Check sheet for the modelled part. Datum: model origin and axes. Units: mm. Coordinates: 2 decimals unless noted, no trailing zeros. Loops run counter-clockwise (first coordinate to the right, second up) from the corner with the lowest first, then second, coordinate; pieces in that order, holes last. Notation, with made-up numbers: M 80.5,75.5 L 93.5,75.5 A33 ccw 93.5,108.5 Z; hole C -17,-22 d10. An arc over 180 degrees is marked long. Use CSV: the item, a comma, the result in double quotes. Start each with the question number.
(1) Go/stop test with flat-tipped pins: pin 1 Ø12 at (y, z) = (-21.5, 27) entering from -X; pin 2 Ø4 at (x, y) = (-55, -19.5) entering from -Z; pin 3 Ø8 at (y, z) = (-11, 32.5) entering from +X. Record where each tip stops, or that it passes through.
(2) Section check C-C on z = 41. Record the cut outline in (x, y), and give its area (3 significant figures).
(3) Section check D-D on y = -23. Record the cut outline in (x, z), and give its area (3 significant figures).
(4) Section check B-B on x = -51. Record the cut outline in (y, z), and give its area (3 significant figures).
(5) Scan lines: line 1 (Z direction, x = -48, y = -13); line 2 (X direction, y = -12.75, z = 47); line 3 (Z direction, x = -43, y = -11). Record each from-to range of solid material in increasing order.
(6) Section check A-A on x = -37.5. Record the cut outline in (y, z), and give its area (3 significant figures).
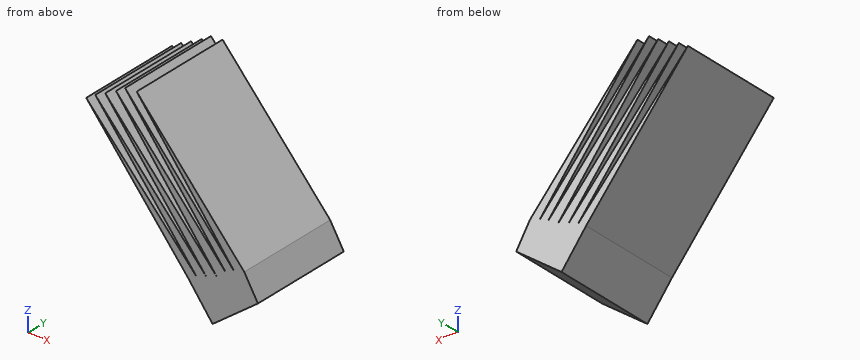
from build123d import *

# Parameters (mm, degrees)
F1_DEPTH = 25.4
F2_DEPTH = 25.4


with BuildPart() as f1:
    # F0 (on Front) → F1 (new body)
    with BuildSketch(Plane.XZ):
        Polygon((-59.2448, 50.682843), (-35.03513, 20.962032), (-29.193482, 13.1901), (-18.408047, 21.296799), (-21.650923, 26.866825), (-47.238376, 56.193985), (-23.816016, 25.882695), (-49.993947, 55.997163), (-25.78428, 24.898561), (-52.159041, 54.619372), (-28.1462, 23.520775), (-54.717787, 53.241584), (-30.704945, 22.733469), (-57.079706, 52.060626), (-32.870036, 21.749334), align=None)
    extrude(amount=F1_DEPTH)

    # F0 (on Front) → F2 (join)
    with BuildSketch(Plane.XZ):
        Polygon((-59.2448, 50.682843), (-35.03513, 20.962032), (-29.193482, 13.1901), (-18.408047, 21.296799), (-21.650923, 26.866825), (-47.238376, 56.193985), (-23.816016, 25.882695), (-49.993947, 55.997163), (-25.78428, 24.898561), (-52.159041, 54.619372), (-28.1462, 23.520775), (-54.717787, 53.241584), (-30.704945, 22.733469), (-57.079706, 52.060626), (-32.870036, 21.749334), align=None)
    extrude(amount=F2_DEPTH)


solid = f1.part
Outcome:
1,pin 1,"stops at x = -44.84"
1,pin 2,"stops at z = 43.02"
1,pin 3,"stops at x = -23.08"
2,outline,"M -51.36,-25.4 L -50.42,-25.4 L -50.42,0 L -51.36,0 Z; M -48.25,-25.4 L -47.13,-25.4 L -47.13,0 L -48.25,0 Z; M -45.08,-25.4 L -43.77,-25.4 L -43.77,0 L -45.08,0 Z; M -41.64,-25.4 L -40.07,-25.4 L -40.07,0 L -41.64,0 Z; M -38.32,-25.4 L -36.96,-25.4 L -36.96,0 L -38.32,0 Z; M -35.5,-25.4 L -33.98,-25.4 L -33.98,0 L -35.5,0 Z"
2,area,"198 mm²"
3,outline,"M -59.24,50.68 L -35.04,20.96 L -29.19,13.19 L -18.41,21.3 L -21.65,26.87 L -47.24,56.19 L -23.82,25.88 L -49.99,56 L -25.78,24.9 L -52.16,54.62 L -28.15,23.52 L -54.72,53.24 L -30.7,22.73 L -57.08,52.06 L -32.87,21.75 Z"
3,area,"385 mm²"
4,outline,"M -25.4,40.56 L 0,40.56 L 0,41.64 L -25.4,41.64 Z; M -25.4,44.45 L 0,44.45 L 0,45.3 L -25.4,45.3 Z; M -25.4,48.52 L 0,48.52 L 0,49.08 L -25.4,49.08 Z; M -25.4,53.12 L 0,53.12 L 0,53.31 L -25.4,53.31 Z"
4,area,"68.3 mm²"
5,line 1,"z = 36.88 to 38.35, 40.69 to 41.96, 44.71 to 45.73, 49.23 to 49.93, 53.44 to 53.7"
5,line 2,"x = -56.24 to -55.89, -53.04 to -52.53, -49.81 to -49.14, -46.28 to -45.4, -42.99 to -42.17, -40.13 to -39.22"
5,line 3,"z = 30.74 to 32.86, 34.43 to 36.4, 38.35 to 40.14, 42.76 to 44.3, 47.01 to 47.95, 50.71 to 51.34"
6,outline,"M -25.4,23.99 L 0,23.99 L 0,26.83 L -25.4,26.83 Z; M -25.4,27.55 L 0,27.55 L 0,30.29 L -25.4,30.29 Z; M -25.4,31.37 L 0,31.37 L 0,33.98 L -25.4,33.98 Z; M -25.4,35.63 L 0,35.63 L 0,38.1 L -25.4,38.1 Z; M -25.4,39.95 L 0,39.95 L 0,41.62 L -25.4,41.62 Z; M -25.4,43.59 L 0,43.59 L 0,45.03 L -25.4,45.03 Z"
6,area,"350 mm²"
